from build123d import *

# Parameters (mm, degrees)
BOSS_EXTRUDE1_DEPTH       = 12
M5X0_8_TAPPED_HOLE1_D     = 4.2
M5X0_8_TAPPED_HOLE1_DEPTH = 14
M5X0_8_TAPPED_HOLE1_TIP   = 1.2618073
M5X0_8_TAPPED_HOLE2_D     = 4.2
M5X0_8_TAPPED_HOLE2_DEPTH = 14
M5X0_8_TAPPED_HOLE2_TIP   = 1.2618073


with BuildPart() as part:
    # Sketch1 → Boss-Extrude1 (new body)
    with BuildSketch(Plane.XY):
        Polygon((0, 75), (5, 80), (20, 80), (20, 3), (17, 0), (0, 0), align=None)
    extrude(amount=BOSS_EXTRUDE1_DEPTH)

    # M5x0.8 Tapped Hole1
    with Locations(Plane.XZ):
        with Locations((8, 6)):
            Hole(M5X0_8_TAPPED_HOLE1_D / 2, depth=M5X0_8_TAPPED_HOLE1_DEPTH)
            with Locations((0, 0, -(M5X0_8_TAPPED_HOLE1_DEPTH + M5X0_8_TAPPED_HOLE1_TIP / 2))):  # 118° drill point
                Cone(0, M5X0_8_TAPPED_HOLE1_D / 2, M5X0_8_TAPPED_HOLE1_TIP, mode=Mode.SUBTRACT)

    # M5x0.8 Tapped Hole2
    with Locations(Plane(origin=(20, 0, 0), x_dir=(0, 0, -1), z_dir=(1, 0, 0))):
        with Locations((-6, 18.5), (-6, 61.5)):
            Hole(M5X0_8_TAPPED_HOLE2_D / 2, depth=M5X0_8_TAPPED_HOLE2_DEPTH)
            with Locations((0, 0, -(M5X0_8_TAPPED_HOLE2_DEPTH + M5X0_8_TAPPED_HOLE2_TIP / 2))):  # 118° drill point
                Cone(0, M5X0_8_TAPPED_HOLE2_D / 2, M5X0_8_TAPPED_HOLE2_TIP, mode=Mode.SUBTRACT)


solid = part.part
Work out the finished part from the listing and answer in its coordinate system (mm). A direction names the side the tool comes from. Round coordinates to 2 decimals unless told otherwise and drop trailing zeros. Loops run counter-clockwise (first coordinate to the right, second up) from the corner with the lowest first, then second, coordinate; pieces in that order, holes last. Notation, with made-up numbers: (53, 12) - (57, 12) arc R17 ccw to (57, 19) - close; hole circle Ø7 at (-3.75, 58). An arc over 180 degrees is marked (long way). Use one line per item in the form item = value. Start each with the question number.
(1) Which of the six approach directions +Z, -Z, +X, -X, +Y, -Y give full straight-line access (tool end or side, diameter ignored) to faces 4 (the face through (12.902, 60.222, 4.334)), 5 (the face through (19, 2, 6)), 6 (the face through (9.548, 7.098, 7.419))?
(2) Determine the mould class of faces 1 (the face through (10, 41, 12)), 2 (the face through (12.9, 20.27, 7.13)), 3 (the face through (20, 42, 6)) for opening direction Z: +Z half, -Z half, draft (parallel to the pull), parting line (faces both ways), or undercut.
(3) Find section B-B on x = 1.75. Determine the outline of the cut face in (y, z), and give its area (3 significant figures).
(4) Find section A-A on x = 18.5. Determine the outline of the cut face in (y, z).
(5) Find section C-C on x = 15. Determine the outline of the cut face in (y, z).
(6) Consider line 1 (Z direction, x = 10, y = 61.5); line 2 (Y direction, x = 15.5, z = 7.25); line 3 (X direction, y = 4.5, z = 6). Determine where each line is inside the solid, lowest interval first.
(7) Flat-ended cylindrical pins translate along their axes: P1, Ø3.5, axis at x = 8, z = 6, coming from the -Y side; P2, Ø4, axis at y = 61.5, z = 6, coming from the +X side; P3, Ø2.5, axis at y = 18.5, z = 6, coming from the +X side. Find the tip coordinate at first contact, or state that the pin passes through.
Answer list:
q1.face_4 = +X
q1.face_5 = +Z, -Z, +X, -Y
q1.face_6 = -Y
q2.face_1 = +Z half
q2.face_2 = undercut
q2.face_3 = draft
q3.outline = (0, 0) - (76.75, 0) - (76.75, 12) - (0, 12) - close
q3.area = 921 mm^2
q4.outline = (1.5, 0) - (80, 0) - (80, 12) - (1.5, 12) - close; hole circle Ø4.2 at (18.5, 6); hole circle Ø4.2 at (61.5, 6)
q5.outline = (0, 0) - (80, 0) - (80, 12) - (0, 12) - close; hole circle Ø4.2 at (18.5, 6); hole circle Ø4.2 at (61.5, 6)
q6.line_1 = 0 to 3.9, 8.1 to 12
q6.line_2 = 0 to 16.81, 20.19 to 59.81, 63.19 to 80
q6.line_3 = 0 to 5.9, 10.1 to 20
q7.P1 = 14.21
q7.P2 = 5.94
q7.P3 = 5.49
